The drawing under review shows one solid part. Ordinate dimensions are in mm from its lowest x, y, z. Coordinates: 2 decimals unless noted, no trailing zeros. Write each loop counter-clockwise with the first axis right and the second up, starting at its lowest first coordinate (ties: lowest second). Pieces come first, ordered by that corner, then holes.
Q1. The part is to be moulded in two halves that separate along X. For the marked faces 1, 2 and 3, say which applies: +X half, -X half, draft (parallel to the pull), parting line (faces both ways), or undercut.
Q2. Add section A-A, the plane x = 12.5. Give the boundary of the cut face in (y, z), plus the area to 3 significant figures.
Q3. Clearance check with flat-ended pins moving along their axes: pin 1 Ø6 at (x, y) = (20, 7) entering from -Z; pin 2 Ø4 at (y, z) = (3, 5.5) entering from -X. State where each tip first meets the part, or that it passes through.
Q4. To check wall thickness, follow probe 1 along X at (y, z) = (5.25, 12.5); probe 2 along X at (y, z) = (7, 15.5); probe 3 along Z at (x, y) = (13, 4.5). State the ranges of each line that lie inside material, in increasing order.
Q5. Add section C-C, the plane y = 3. Give the boundary of the cut face in (x, z).
Q6. Add section B-B, the plane z = 12.5. Give the boundary of the cut face in (x, y).
Q7. Add section D-D, the plane y = 7.75. Give the boundary of the cut face in (x, z).
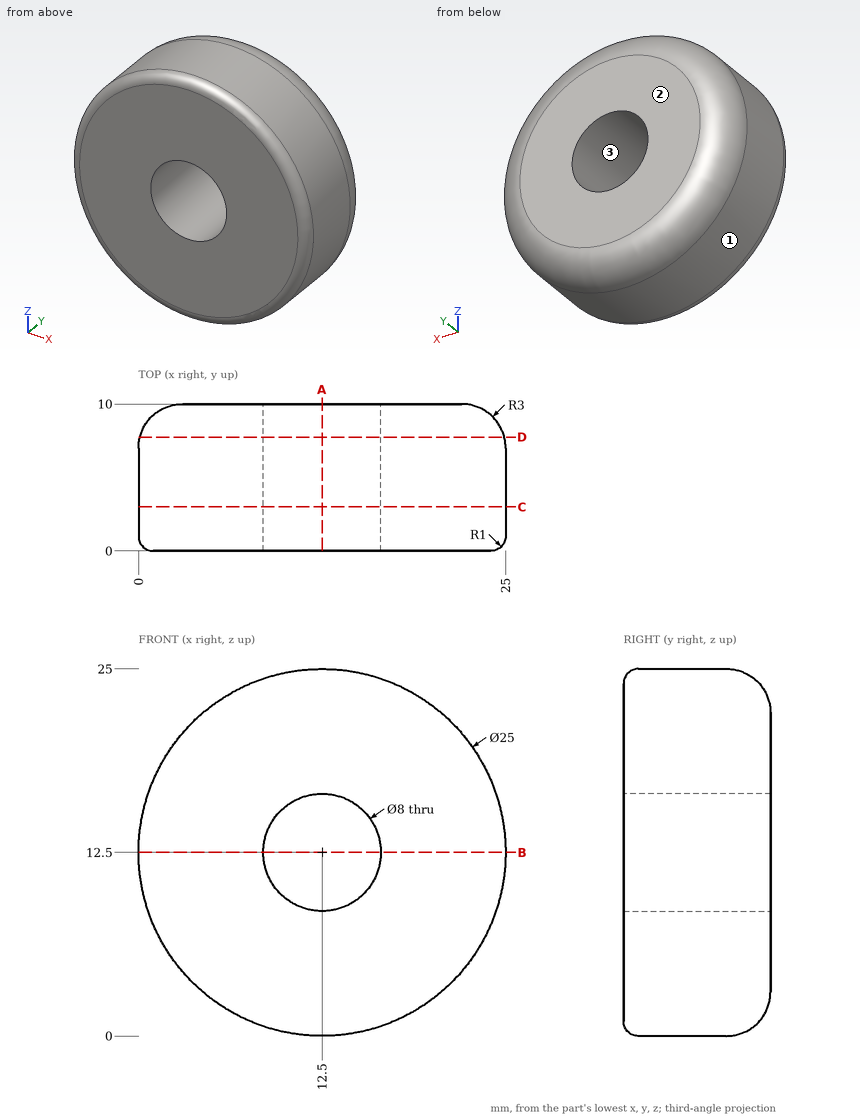
Here are the results:
1. face 1: parting line
1. face 2: draft
1. face 3: undercut
2. outline: (0, 1) arc R1 ccw to (1, 0) - (7, 0) arc R3 ccw to (10, 3) - (10, 8.5) - (0, 8.5) - close; (0, 16.5) - (10, 16.5) - (10, 22) arc R3 ccw to (7, 25) - (1, 25) arc R1 ccw to (0, 24) - close
2. area: 166 mm2
3. pin 1: stops at z = 0.84
3. pin 2: stops at x = 1.04
4. probe 1: x = 0 to 8.5, 16.5 to 25
4. probe 2: x = 0.37 to 9.85, 15.15 to 24.63
4. probe 3: z = 0.01 to 8.53, 16.47 to 24.99
5. outline: circle Ø25 at (12.5, 12.5); hole circle Ø8 at (12.5, 12.5)
6. outline: (0, 1) arc R1 ccw to (1, 0) - (8.5, 0) - (8.5, 10) - (3, 10) arc R3 ccw to (0, 7) - close; (16.5, 0) - (24, 0) arc R1 ccw to (25, 1) - (25, 7) arc R3 ccw to (22, 10) - (16.5, 10) - close
7. outline: circle Ø24.81 at (12.5, 12.5); hole circle Ø8 at (12.5, 12.5)
